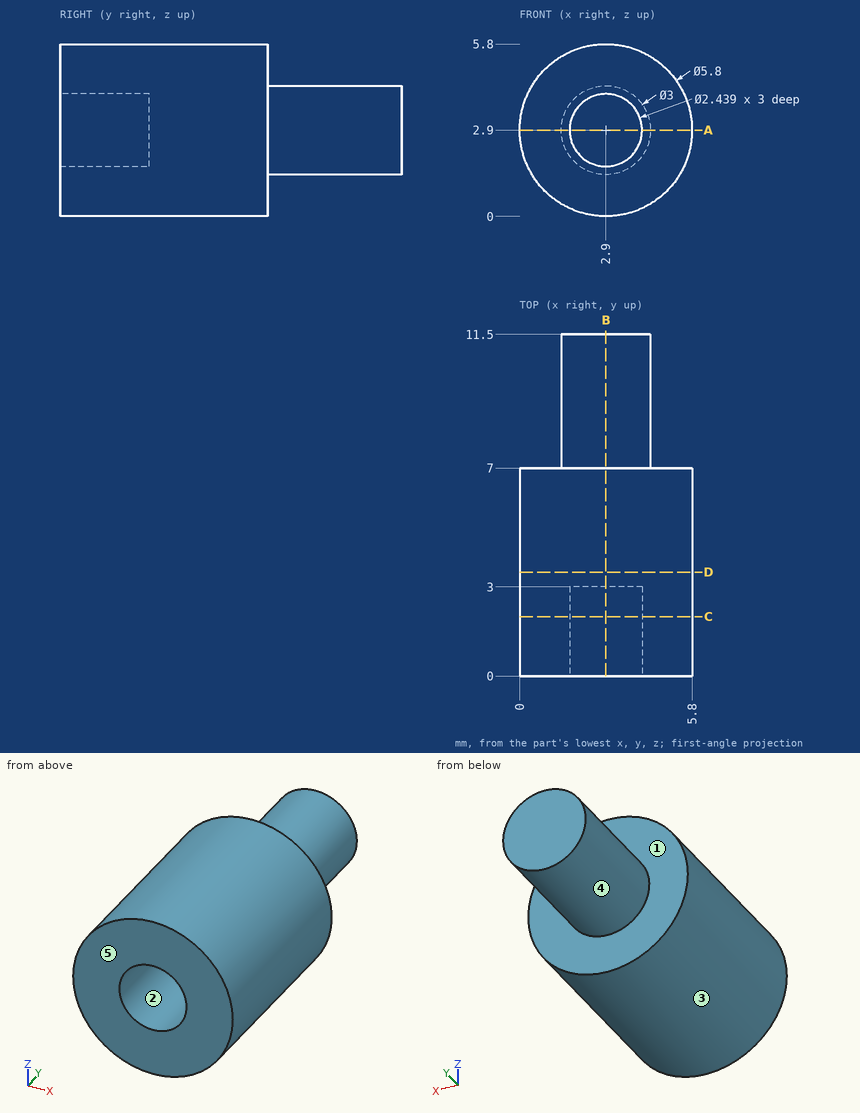
Input: dimensioned drawing with shaded views. Units: mm. Origin: part minimum x, y, z. A direction names the side the tool comes from. Round coordinates to 2 decimals unless told otherwise and drop trailing zeros. Write each loop counter-clockwise with the first axis right and the second up, starting at its lowest first coordinate (ties: lowest second). Pieces come first, ordered by that corner, then holes. Notation, with made-up numbers: (-34, 1) -> (18, 1) arc R24 ccw to (18, 19) -> close; hole circle Ø3 at (-34, 50.25). An arc over 180 degrees is marked (long way). Use CSV: the item, a comma, the result in double quotes. Start each with the question number.
Q1. Reachability of the marked faces 4 and 5 from +Z, -Z, +X, -X, +Y, -Y: full face, straight path, thin tool, end or side. Return the list, or none.
Q2. Section A-A (z = 2.9). Return loops of the section in (x, y), plus the area to 3 significant figures.
Q3. Pull-direction query (X, two-part tool) for the marked faces 1, 2 and 3; classes: pulls with the +X half, pulls with the -X half, needs draft (parallel to the pull), parting line crosses it, or undercut.
Q4. Section B-B (x = 2.9). Return loops of the section in (y, z).
Q5. Line query: L1, parallel to X at y = 2.4, z = 2.9; L2, parallel to Y at x = 4.55, z = 2.1. Output: solid intervals per line, ascending.
Q6. Section C-C (y = 2). Return loops of the section in (x, z).
Q7. Section D-D (y = 3.5). Return loops of the section in (x, z), plus the area to 3 significant figures.
Q8. First-contact query: pin 1 Ø0.7 at (x, z) = (2.5, 3) entering from -Y; pin 2 Ø1.5 at (x, y) = (0.5, 8) entering from -Z; pin 3 Ø1.5 at (x, y) = (1.5, 7) entering from +Z; pin 4 Ø2 at (x, y) = (4.5, 9.5) entering from +Z. Flat tips, straight axial feed; report the tip coordinate or a pass-through.
Result sheet:
1,face 4,"+Y"
1,face 5,"+Z, -Z, +X, -X, -Y"
2,outline,"(0, 0) -> (1.68, 0) -> (1.68, 3) -> (4.12, 3) -> (4.12, 0) -> (5.8, 0) -> (5.8, 7) -> (4.4, 7) -> (4.4, 11.5) -> (1.4, 11.5) -> (1.4, 7) -> (0, 7) -> close"
2,area,"46.8 mm²"
3,face 1,"needs draft"
3,face 2,"undercut"
3,face 3,"parting line crosses it"
4,outline,"(0, 0) -> (7, 0) -> (7, 1.4) -> (11.5, 1.4) -> (11.5, 4.4) -> (7, 4.4) -> (7, 5.8) -> (0, 5.8) -> (0, 4.12) -> (3, 4.12) -> (3, 1.68) -> (0, 1.68) -> close"
5,L1,"0 to 1.68, 4.12 to 5.8"
5,L2,"0 to 7"
6,outline,"circle Ø5.8 at (2.9, 2.9); hole circle Ø2.44 at (2.9, 2.9)"
7,outline,"circle Ø5.8 at (2.9, 2.9)"
7,area,"26.4 mm²"
8,pin 1,"y = 3"
8,pin 2,"through"
8,pin 3,"z = 5.73"
8,pin 4,"z = 4.27"
